from build123d import *

# Parameters (mm, degrees)
SKETCH_1_R          = 24.5
EXTRUDE_1_DEPTH     = 12.5
SKETCH_2_R          = 1.25
CUT_EXTRUDE_1_DEPTH = 3
SKETCH_3_R          = 1.5
CUT_EXTRUDE_2_DEPTH = 3.5
SKETCH_5_R          = 6.35
CUT_EXTRUDE_3_DEPTH = 10


with BuildPart() as part:
    # 草图1 → 凸台-拉伸1 (new body)
    with BuildSketch(Plane.XY):
        Circle(SKETCH_1_R)
    extrude(amount=EXTRUDE_1_DEPTH)

    # 草图2 → 切除-拉伸1 (cut)
    with BuildSketch(Plane.XY.offset(12.5)):
        with Locations((0, 22)):
            Circle(SKETCH_2_R)
        with Locations((0, -22)):
            Circle(SKETCH_2_R)
        with Locations((19.052558883, 11)):
            Circle(SKETCH_2_R)
        with Locations((-19.052558883, 11)):
            Circle(SKETCH_2_R)
        with Locations((19.052558883, -11)):
            Circle(SKETCH_2_R)
        with Locations((-19.052558883, -11)):
            Circle(SKETCH_2_R)
    extrude(amount=-CUT_EXTRUDE_1_DEPTH, mode=Mode.SUBTRACT)

    # 草图3 → 切除-拉伸2 (cut)
    with BuildSketch(Plane.XY.offset(12.5)):
        with Locations((0, 12.5)):
            Circle(SKETCH_3_R)
        with Locations((0, -12.5)):
            Circle(SKETCH_3_R)
        with Locations((12.5, 0)):
            Circle(SKETCH_3_R)
        with Locations((-12.5, 0)):
            Circle(SKETCH_3_R)
    extrude(amount=-CUT_EXTRUDE_2_DEPTH, mode=Mode.SUBTRACT)

    # 草图5 → 切除-拉伸3 (cut)
    with BuildSketch(Plane.XY.offset(12.5)):
        Circle(SKETCH_5_R)
    extrude(amount=-CUT_EXTRUDE_3_DEPTH, mode=Mode.SUBTRACT)


solid = part.part
Build history of the part. All positions in model axes, mm. Give positions to 0.01 mm unless a question says otherwise; leave off trailing zeros. Order: outer loops, then holes, each group sorted by start corner. A loop starts at its lowest first (then second) coordinate and runs counter-clockwise, first axis right, second up. Notation, with made-up numbers: M -17.75,-29 L 35.25,-29 A25 cw 35.25,-8 Z; hole C 82.25,2.25 d3. An arc over 180 degrees is marked long. Put each result on its own line as item: value.
Item 1: Flat gauge pins, fed straight in: pin 1 Ø2 at (x, y) = (0, -22) entering from +Z; pin 2 Ø3.5 at (x, y) = (12, 0) entering from +Z; pin 3 Ø1.5 at (y, z) = (-2, 9.5) entering from -X; pin 4 Ø2.5 at (x, y) = (0, -12.5) entering from +Z. Where does each tip first touch, or does it go through?
From the geometry:
pin 1: stops at z = 9.5
pin 2: stops at z = 12.5
pin 3: stops at x = -24.47
pin 4: stops at z = 9
Item 2: Slice it at C-C, the plane x = -5.5. Write the cut outline in (y, z), plus the area to 3 significant figures.
From the geometry:
outline: M -23.87,0 L 23.87,0 L 23.87,12.5 L 3.17,12.5 L 3.17,2.5 L -3.17,2.5 L -3.17,12.5 L -23.87,12.5 Z
area: 533 mm2
Item 3: Two-plate mould, pull along Y, no slides. Class faces 1 (the flat face through (5, -5, 12.5)), 2 (the cylindrical face through (-0.27, -23.22, 11.02)): +Y half, -Y half, draft (parallel to the pull), parting line (faces both ways), or undercut.
From the geometry:
face 1: draft
face 2: undercut
Item 4: Slice it at A-A, the plane z = 11.75. Give the number of separate pieces and of enclosed holes in the cut face, plus the area to 3 significant figures.
From the geometry:
separate pieces: 1
enclosed holes: 11
area: 1,700 mm2
Item 5: Probe line 1 (Y direction, x = 0, z = 10.35); line 2 (Y direction, x = 12.5, z = 9.95); line 3 (X direction, y = 2, z = 3.5). List the from-to ranges inside material, lowest first. Write a range as [from, to].
From the geometry:
line 1: y = [-24.5, -23.25], [-20.75, -14], [-11, -6.35], [6.35, 11], [14, 20.75], [23.25, 24.5]
line 2: y = [-21.07, -1.5], [1.5, 21.07]
line 3: x = [-24.42, -6.03], [6.03, 24.42]
Item 6: Slice it at D-D, the plane y = 22. Write the cut outline in (x, z), plus the area to 3 significant figures.
From the geometry:
outline: M -10.78,0 L 10.78,0 L 10.78,12.5 L 1.25,12.5 L 1.25,9.5 L -1.25,9.5 L -1.25,12.5 L -10.78,12.5 Z
area: 262 mm2
Item 7: Slice it at B-B, the plane z = 5.5. Write the cut outline in (x, y).
From the geometry:
outline: C 0,0 d49; hole C 0,0 d12.7
